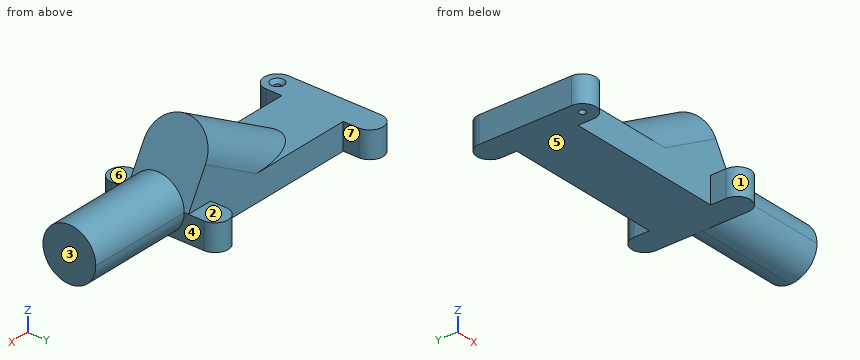
from build123d import *

# Parameters (mm, degrees)
F1_DEPTH        = 25.4
F6_DEPTH        = 101.6
F10_D           = 6.35
F10_CSINK_D     = 12.7
F10_CSINK_ANGLE = 90


with BuildPart() as f1:
    # F0 (on Top) → F1 (new body)
    with BuildSketch(Plane.XY):
        with BuildLine():
            Line((0, -59.0296), (0, 0))
            Line((0, 0), (-76.2, 0))
            Line((-76.2, 0), (-76.2, 14.9352))
            ThreePointArc((-76.2, 14.9352), (-88.9, 27.6352), (-101.6, 14.9352))
            Line((-101.6, 14.9352), (-101.6, -73.9648))
            ThreePointArc((-101.6, -73.9648), (-88.9, -86.6648), (-76.2, -73.9648))
            Line((-76.2, -73.9648), (-76.2, -59.0296))
            Line((-76.2, -59.0296), (0, -59.0296))
        make_face()
        with BuildLine():
            Line((76.2, 0), (0, 0))
            Line((0, 0), (0, -59.0296))
            Line((0, -59.0296), (76.2, -59.0296))
            Line((76.2, -59.0296), (76.2, -73.9648))
            ThreePointArc((76.2, -73.9648), (88.9, -86.6648), (101.6, -73.9648))
            Line((101.6, -73.9648), (101.6, 14.9352))
            ThreePointArc((101.6, 14.9352), (88.9, 27.6352), (76.2, 14.9352))
            Line((76.2, 14.9352), (76.2, 0))
        make_face()
    extrude(amount=F1_DEPTH)

    # F3 (on face) → F4 (join, up to the next surface of F1)
    with BuildSketch(Plane(origin=(87.1985226281, 0, 50.3440905122), x_dir=(0, 1, 0), z_dir=(0.8660254038, 0, 0.5))):
        with BuildLine():
            Line((-59.0296, 10.1618718698), (-59.0296, -28.8029547439))
            Line((-59.0296, -28.8029547439), (0, -28.8029547439))
            Line((0, -28.8029547439), (0, 10.1618718698))
            ThreePointArc((0, 10.1618718698), (-29.5148, 39.6766718698), (-59.0296, 10.1618718698))
        make_face()
    extrude(until=Until.NEXT, dir=(-0.8660254038, 0, -0.5))

    # F5 (on face) → F6 (join)
    with BuildSketch(Plane.YZ.offset(101.6)):
        with BuildLine():
            Line((-54.9148, 25.4), (-4.1148, 25.4))
            ThreePointArc((-4.1148, 25.4), (-29.5148, 50.8), (-54.9148, 25.4))
        make_face()
        with BuildLine():
            ThreePointArc((-29.5148, 0), (-11.5542877579, 7.4394877579), (-4.1148, 25.4))
            Line((-4.1148, 25.4), (-54.9148, 25.4))
            ThreePointArc((-54.9148, 25.4), (-47.4753122421, 7.4394877579), (-29.5148, 0))
        make_face()
    extrude(amount=F6_DEPTH)

    # F10 (through all)
    with Locations(Plane.XY.offset(25.4)):
        with Locations((-88.9, -73.9648)):
            CounterSinkHole(F10_D / 2, F10_CSINK_D / 2, counter_sink_angle=F10_CSINK_ANGLE)


solid = f1.part
Build history of the part. All positions in model axes, mm. Face numbers are marked on the shaded views. A direction names the side the tool comes from. Round coordinates to 2 decimals unless told otherwise and drop trailing zeros. Loops run counter-clockwise (first coordinate to the right, second up) from the corner with the lowest first, then second, coordinate; pieces in that order, holes last. Notation, with made-up numbers: (0, -18.5) -> (18, -18.5) arc R20 cw to (18, -13.5) -> close; hole circle Ø4 at (69.5, 64). An arc over 180 degrees is marked (long way). Answer in a Markdown table with one row per item.
Item 1: Saw through at D-D (y = -36). Write the cut outline in (x, z), and give its area (3 significant figures).
Answers below:
| item | result |
|---|---|
| outline | (-101.6, 0) -> (101.6, 0) -> (101.6, 0.84) -> (203.2, 0.84) -> (203.2, 49.96) -> (101.6, 49.96) -> (101.6, 25.4) -> (67.72, 84.08) -> (-33.92, 25.4) -> (-101.6, 25.4) -> close |
| area | 14,100 mm² |
Item 2: Which spindle directions (+Z, -Z, +X, -X, +Y, -Y) get a long thin tool onto all of the face, cutting with end or side? Do the marked faces 4, 5, 6 and 7. Say none if no direction does.
Answers below:
| item | result |
|---|---|
| face 4 | -Z, +X, +Y |
| face 5 | -Z, +X, -X, +Y, -Y |
| face 6 | +Z, +X, -X, -Y |
| face 7 | +Z, -Z, +Y |
Item 3: Pin check, flat tips, straight feed: pin 1 (17.5 mm diameter, centred on x = 29, z = 35, fed in from -Y); pin 2 (8 mm diameter, centred on x = 169, y = -27.5, fed in from -Z); pin 3 (8 mm diameter, centred on x = 164.5, y = -41.5, fed in from -Z); pin 4 (1 mm diameter, centred on y = 8, z = 17, fed in from +X). Stop position of each tip, or through.
Answers below:
| item | result |
|---|---|
| pin 1 | stops at y = -59.03 |
| pin 2 | stops at z = 0 |
| pin 3 | stops at z = 1.29 |
| pin 4 | stops at x = 101.6 |
Item 4: Saw through at B-B (x = -88.9). Write the cut outline in (y, z) (3 decimals).
Answers below:
| item | result |
|---|---|
| outline | (-86.665, 0) -> (-77.14, 0) -> (-77.14, 22.225) -> (-80.315, 25.4) -> (-86.665, 25.4) -> close; (-70.79, 0) -> (27.635, 0) -> (27.635, 25.4) -> (-67.615, 25.4) -> (-70.79, 22.225) -> close |
Item 5: Saw through at A-A (y = -64). Write the cut outline in (x, z).
Answers below:
| item | result |
|---|---|
| outline | (-101.6, 0) -> (-76.2, 0) -> (-76.2, 25.4) -> (-101.6, 25.4) -> close; (76.2, 0) -> (101.6, 0) -> (101.6, 25.4) -> (76.2, 25.4) -> close |
Item 6: Mould opens along X. For the marked faces 1, 2 and 3 say: +X half, -X half, draft (parallel to the pull), parting line (faces both ways), or undercut.
Answers below:
| item | result |
|---|---|
| face 1 | undercut |
| face 2 | draft |
| face 3 | +X half |
Item 7: Drill centre lines: L1, parallel to X at y = -61.5, z = 4; L2, parallel to Y at x = -88, z = 6; L3, parallel to Y at x = -88.9, z = 5.5. Where is each one in solid material? Low to high. Write a range as [from, to].
Answers below:
| item | result |
|---|---|
| L1 | x = [-101.6, -76.2], [76.2, 101.6] |
| L2 | y = [-86.63, -77.01], [-70.92, 27.6] |
| L3 | y = [-86.66, -77.14], [-70.79, 27.64] |
Item 8: Saw through at C-C (z = 8). Write the cut outline in (x, y) (3 decimals), and give its area (3 significant figures).
Answers below:
| item | result |
|---|---|
| outline | (-101.6, -73.965) arc R12.7 ccw to (-76.2, -73.965) -> (-76.2, -59.03) -> (76.2, -59.03) -> (76.2, -73.965) arc R12.7 ccw to (101.6, -73.965) -> (101.6, -48.019) -> (203.2, -48.019) -> (203.2, -11.011) -> (101.6, -11.011) -> (101.6, 14.935) arc R12.7 ccw to (76.2, 14.935) -> (76.2, 0) -> (-76.2, 0) -> (-76.2, 14.935) arc R12.7 ccw to (-101.6, 14.935) -> close; hole circle Ø6.35 at (-88.9, -73.965) |
| area | 18,300 mm² |
